The drawing under review shows one solid part. Ordinate dimensions are in mm from its lowest x, y, z. A direction names the side the tool comes from. Round coordinates to 2 decimals unless told otherwise and drop trailing zeros. Write each loop counter-clockwise with the first axis right and the second up, starting at its lowest first coordinate (ties: lowest second). Pieces come first, ordered by that corner, then holes. Notation, with made-up numbers: (-24.5, 48) -> (15.5, 48) arc R31 cw to (15.5, 77) -> close; hole circle Ø4 at (-28, 48). An arc over 180 degrees is marked (long way). Write item = value, one per line. Start each with the question number.
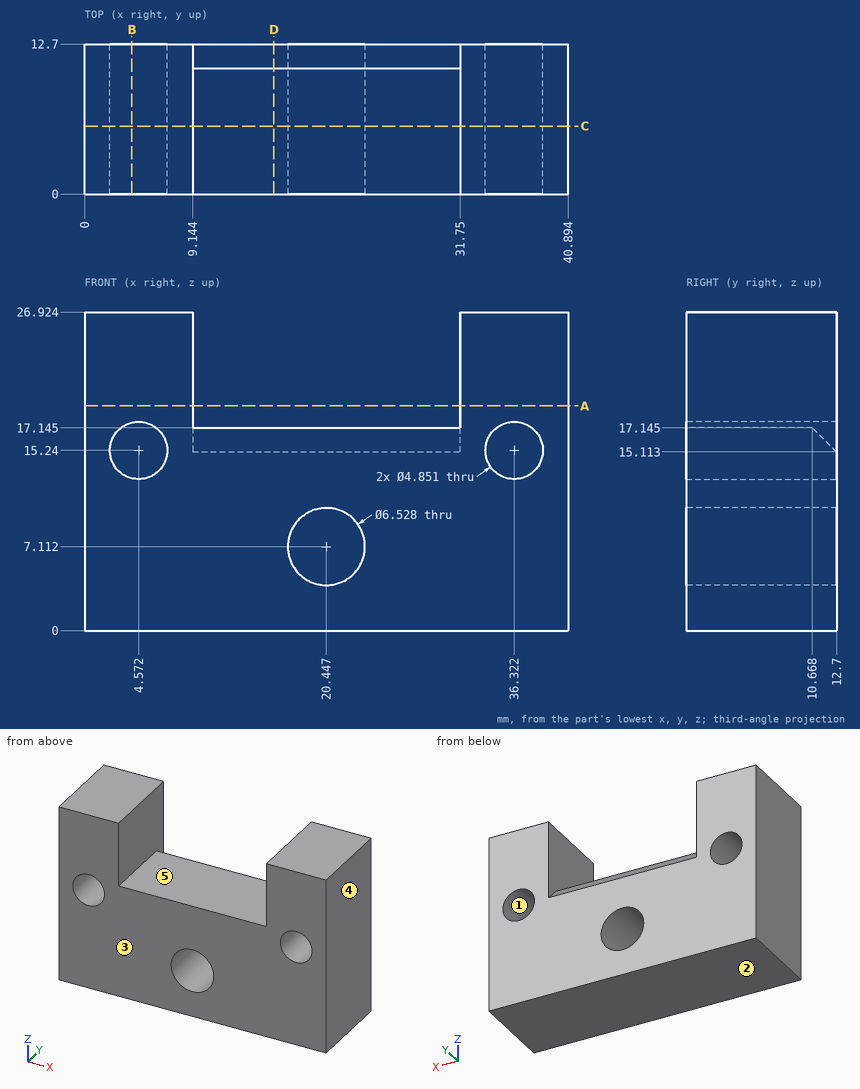
1. Wall thickness on L1, parallel to X at y = 4, z = 15.24; L2, parallel to X at y = 4.25, z = 7.25; L3, parallel to Z at x = 36.5, y = 7.5: over which ranges is each line inside the solid? List them lowest first. Write a range as from..to.
2. Consider section D-D, the plane x = 16. Give the boundary of the cut face in (y, z) (1 decimal).
3. Machinability: for the marked faces 4 and 5, which of the approach directions +Z, -Z, +X, -X, +Y, -Y give a long, thin tool a straight path to every point of the face, cutting with its end or side? Answer none if there is none.
4. Clearance check with flat-ended pins moving along their axes: pin 1 Ø3 at (x, y) = (17.5, 4) entering from +Z (3 decimals); pin 2 Ø4.5 at (x, z) = (4.572, 15.24) entering from +Y. State where each tip first meets the part, or that it passes through.
5. Draft analysis for pull direction Z (two halves, no side actions). For the marked faces 1, 2 and 3, state which applies: +Z half, -Z half, draft (parallel to the pull), parting line (faces both ways), or undercut.
6. Consider section A-A, the plane z = 19. Give the boundary of the cut face in (x, y).
7. Consider section C-C, the plane y = 5.75. Give the number of separate pieces and of enclosed holes in the cut face.
8. Consider section B-B, the plane x = 4. Give the boundary of the cut face in (y, z).
Outcome:
q1.L1 = 0..2.15, 7..33.9, 38.75..40.89
q1.L2 = 0..17.19, 23.71..40.89
q1.L3 = 0..12.82, 17.66..26.92
q2.outline = (0, 0) -> (12.7, 0) -> (12.7, 15.1) -> (10.7, 17.1) -> (0, 17.1) -> close
q3.face_4 = +Z, -Z, +X, +Y, -Y
q3.face_5 = +Z, +Y, -Y
q4.pin_1 = 17.145
q4.pin_2 = through
q5.face_1 = undercut
q5.face_2 = -Z half
q5.face_3 = draft
q6.outline = (0, 0) -> (9.14, 0) -> (9.14, 12.7) -> (0, 12.7) -> close; (31.75, 0) -> (40.89, 0) -> (40.89, 12.7) -> (31.75, 12.7) -> close
q7.separate_pieces = 1
q7.enclosed_holes = 3
q8.outline = (0, 0) -> (12.7, 0) -> (12.7, 12.88) -> (0, 12.88) -> close; (0, 17.6) -> (12.7, 17.6) -> (12.7, 26.92) -> (0, 26.92) -> close
